Check sheet for the modelled part. Datum: model origin and axes. Units: mm. A direction names the side the tool comes from. Coordinates: 2 decimals unless noted, no trailing zeros. Loops run counter-clockwise (first coordinate to the right, second up) from the corner with the lowest first, then second, coordinate; pieces in that order, holes last. Notation, with made-up numbers: (22.5, 77.25) - (53.5, 77.25) arc R11 ccw to (53.5, 95.25) - close; hole circle Ø4 at (-32.5, -22.75). An arc over 180 degrees is marked (long way). Use a Markdown table: item, result. Add a question column.
1) Thickness scan on line 1 (X direction, y = -1.6, z = 0); line 2 (Y direction, x = 12.5, z = -28); line 3 (X direction, y = -7.5, z = -47.5). Record the ranges inside material, lowest first.
2) Go/stop test with flat-tipped pins: P1, Ø1.5, axis at y = -9, z = 35.5, coming from the -X side; P2, Ø15, axis at x = 4.5, z = -7.5, coming from the +Y side; P3, Ø2, axis at x = 0, z = -31, coming from the -Y side; P4, Ø3, axis at x = -3, z = -26.5, coming from the +Y side. Record where each tip stops, or that it passes through.
3) Draft check along X on faces 4 (the cylindrical face through (52.5, -6.4, 0.1)), 5 (the flat face through (0, -4.555, 30)), 6 (the flat face through (43, -6, -5)). Enter one of: pulls with the +X half, pulls with the -X half, needs draft (parallel to the pull), parting line crosses it, or undercut.
4) Sectioned sample at A-A, the plane y = -7.5. State how many separate pieces and enclosed holes the cut face has, then the cut area to 3 significant figures.
5) Sectioned sample at B-B, the plane x = -30. Enter the section's corners in (y, z).
6) Sectioned sample at C-C, the plane z = -30. Enter the section's corners in (x, y).
7) Tool access check on faces 1 (the flat face through (5, -6, -43)), 2 (the flat face through (24.5, -1.955, -7.8)), 3 (the flat face through (-43, -6, -5)). Record the directions out of +Z, -Z, +X, -X, +Y, -Y that give a thin tool (end or side, any length) a straight path to the whole face; none if there is none.
from build123d import *

# Parameters (mm, degrees)
SKETCH2_R           = 2.15
BOSS_EXTRUDE1_DEPTH = 10.507214
CUT_EXTRUDE2_DEPTH  = 7
SKETCH4_R           = 2.15
CUT_EXTRUDE3_DEPTH  = 7
BOSS_EXTRUDE2_START = -7
SKETCH5_R           = 24.3
SKETCH5_R_2         = 23.3
BOSS_EXTRUDE2_DEPTH = 7
SKETCH6_R           = 23.3
CUT_EXTRUDE4_DEPTH  = 75.575465


with BuildPart() as part:
    # Sketch1 → Revolve1 (revolve)
    with BuildSketch(Plane(origin=(0, 0, 0), x_dir=(0, 0, -1), z_dir=(1, 0, 0)), mode=Mode.PRIVATE) as revolve1_sk:
        with BuildLine():
            Line((-37.5, -1.048229), (-37.5, -1.955443))
            Line((-37.5, -1.955443), (-25.3, -1.955443))
            ThreePointArc((-25.3, -1.955443), (-25, -2.455443), (-25.3, -2.955443))
            Line((-25.3, -2.955443), (-25.3, -4.555443))
            Line((-25.3, -4.555443), (-8, -4.555443))
            Line((-8, -4.555443), (-8, -11.555443))
            Line((-8, -11.555443), (-39.5, -11.555443))
            Line((-39.5, -11.555443), (-39.5, -1.048229))
            Line((-39.5, -1.048229), (-37.5, -1.048229))
        make_face()
    revolve(revolve1_sk.sketch.rotate(Axis((0, -1000, 0), (0, 1, 0)), 180), axis=Axis((0, -1000, 0), (0, 1, 0)))

    # Sketch2 → Boss-Extrude1 (add)
    # profile 1 of 4: a face of its own
    with BuildSketch(Plane.XZ.offset(11.555443)):
        with BuildLine():
            Line((-5, 47.5), (-5, 39.182266))
            Line((-5, 39.182266), (5, 39.182266))
            Line((5, 39.182266), (5, 47.5))
            ThreePointArc((5, 47.5), (0, 52.5), (-5, 47.5))
        make_face()
        with Locations(Location((0, 47.5, 0), (0, 0, 270))):
            Circle(SKETCH2_R, mode=Mode.SUBTRACT)
    # profile 2 of 4: a face of its own
    with BuildSketch(Plane.XZ.offset(11.555443)):
        with BuildLine():
            Line((47.5, -5), (39.182266, -5))
            Line((39.182266, -5), (39.182266, 5))
            Line((39.182266, 5), (47.5, 5))
            ThreePointArc((47.5, 5), (52.5, 0), (47.5, -5))
        make_face()
        with Locations(Location((47.5, 0, 0), (0, 0, 270))):
            Circle(SKETCH2_R, mode=Mode.SUBTRACT)
    # profile 3 of 4: a face of its own
    with BuildSketch(Plane.XZ.offset(11.555443)):
        with BuildLine():
            Line((-5, -47.5), (-5, -39.182266))
            Line((-5, -39.182266), (5, -39.182266))
            Line((5, -39.182266), (5, -47.5))
            ThreePointArc((5, -47.5), (0, -52.5), (-5, -47.5))
        make_face()
        with Locations(Location((0, -47.5, 0), (0, 0, 270))):
            Circle(SKETCH2_R, mode=Mode.SUBTRACT)
    # profile 4 of 4: a face of its own
    with BuildSketch(Plane.XZ.offset(11.555443)):
        with BuildLine():
            Line((-47.5, 5), (-39.182266, 5))
            Line((-39.182266, 5), (-39.182266, -5))
            Line((-39.182266, -5), (-47.5, -5))
            ThreePointArc((-47.5, -5), (-52.5, 0), (-47.5, 5))
        make_face()
        with Locations(Location((-47.5, 0, 0), (0, 0, 270))):
            Circle(SKETCH2_R, mode=Mode.SUBTRACT)
    extrude(amount=-BOSS_EXTRUDE1_DEPTH)

    # Sketch3 → Cut-Extrude2 (cut)
    with BuildSketch(Plane(origin=(0, -4.555443, 0), x_dir=(1, 0, 0), z_dir=(0, 1, 0))):
        with BuildLine():
            Line((21.938323, -2), (12.369317, -2))
            ThreePointArc((12.369317, -2), (11.19262, -2.382785), (10.466345, -3.384615))
            ThreePointArc((10.466345, -3.384615), (7.778175, -7.778175), (3.384615, -10.466345))
            ThreePointArc((3.384615, -10.466345), (2.382785, -11.19262), (2, -12.369317))
            Line((2, -12.369317), (2, -21.938323))
            ThreePointArc((2, -21.938323), (2.718885, -23.474143), (4.358744, -23.905885))
            ThreePointArc((4.358744, -23.905885), (17.182695, -17.182695), (23.905885, -4.358744))
            ThreePointArc((23.905885, -4.358744), (23.474143, -2.718885), (21.938323, -2))
        make_face()
        with BuildLine():
            Line((-2, -21.938323), (-2, -12.369317))
            ThreePointArc((-2, -12.369317), (-2.382785, -11.19262), (-3.384615, -10.466345))
            ThreePointArc((-3.384615, -10.466345), (-7.778175, -7.778175), (-10.466345, -3.384615))
            ThreePointArc((-10.466345, -3.384615), (-11.19262, -2.382785), (-12.369317, -2))
            Line((-12.369317, -2), (-21.938323, -2))
            ThreePointArc((-21.938323, -2), (-23.474143, -2.718885), (-23.905885, -4.358744))
            ThreePointArc((-23.905885, -4.358744), (-17.182695, -17.182695), (-4.358744, -23.905885))
            ThreePointArc((-4.358744, -23.905885), (-2.718885, -23.474143), (-2, -21.938323))
        make_face()
        with BuildLine():
            Line((-21.938323, 2), (-12.369317, 2))
            ThreePointArc((-12.369317, 2), (-11.19262, 2.382785), (-10.466345, 3.384615))
            ThreePointArc((-10.466345, 3.384615), (-7.778175, 7.778175), (-3.384615, 10.466345))
            ThreePointArc((-3.384615, 10.466345), (-2.382785, 11.19262), (-2, 12.369317))
            Line((-2, 12.369317), (-2, 21.938323))
            ThreePointArc((-2, 21.938323), (-2.718885, 23.474143), (-4.358744, 23.905885))
            ThreePointArc((-4.358744, 23.905885), (-17.182695, 17.182695), (-23.905885, 4.358744))
            ThreePointArc((-23.905885, 4.358744), (-23.474143, 2.718885), (-21.938323, 2))
        make_face()
        with BuildLine():
            Line((2, 21.938323), (2, 12.369317))
            ThreePointArc((2, 12.369317), (2.382785, 11.19262), (3.384615, 10.466345))
            ThreePointArc((3.384615, 10.466345), (7.778175, 7.778175), (10.466345, 3.384615))
            ThreePointArc((10.466345, 3.384615), (11.19262, 2.382785), (12.369317, 2))
            Line((12.369317, 2), (21.938323, 2))
            ThreePointArc((21.938323, 2), (23.474143, 2.718885), (23.905885, 4.358744))
            ThreePointArc((23.905885, 4.358744), (17.182695, 17.182695), (4.358744, 23.905885))
            ThreePointArc((4.358744, 23.905885), (2.718885, 23.474143), (2, 21.938323))
        make_face()
    extrude(amount=-CUT_EXTRUDE2_DEPTH, mode=Mode.SUBTRACT)

    # Sketch4 → Cut-Extrude3 (cut)
    with BuildSketch(Plane(origin=(0, -11.555443, 0), x_dir=(-1, 0, 0), z_dir=(0, -1, 0))):
        with Locations(Location((30, 0, 0), (0, 0, 90))):
            Circle(SKETCH4_R)
        with Locations(Location((0, -30, 0), (0, 0, 90))):
            Circle(SKETCH4_R)
        with Locations(Location((-30, 0, 0), (0, 0, 90))):
            Circle(SKETCH4_R)
        with Locations(Location((0, 30, 0), (0, 0, 90))):
            Circle(SKETCH4_R)
    extrude(amount=-CUT_EXTRUDE3_DEPTH, mode=Mode.SUBTRACT)

    # Sketch5 → Boss-Extrude2 (add)
    with BuildSketch(Plane.XZ.offset(11.555443).offset(BOSS_EXTRUDE2_START)):
        Circle(SKETCH5_R)
        Circle(SKETCH5_R_2, mode=Mode.SUBTRACT)
    extrude(amount=BOSS_EXTRUDE2_DEPTH)

    # Sketch6 → Cut-Extrude4 (cut, through all)
    with BuildSketch(Plane(origin=(0, -4.555443, 0), x_dir=(1, 0, 0), z_dir=(0, 1, 0))):
        with Locations(Location((0, 0, 0), (0, 0, 90))):
            Circle(SKETCH6_R)
    extrude(amount=-CUT_EXTRUDE4_DEPTH, mode=Mode.SUBTRACT)


solid = part.part
Solved:
| question | item | result |
|---|---|---|
| 1 | line 1 | x = -52.5 to -49.65, -45.35 to -37.5, 37.5 to 45.35, 49.65 to 52.5 |
| 1 | line 2 | y = -11.56 to -1.96 |
| 1 | line 3 | x = -5 to -2.15, 2.15 to 5 |
| 2 | P1 | stops at x = -18.78 |
| 2 | P2 | passes through |
| 2 | P3 | stops at y = -4.56 |
| 2 | P4 | stops at y = -1.96 |
| 3 | face 4 | pulls with the +X half |
| 3 | face 5 | undercut |
| 3 | face 6 | needs draft |
| 4 | separate pieces | 1 |
| 4 | enclosed holes | 9 |
| 4 | area | 3,560 mm2 |
| 5 | outline | (-11.56, -25.7) - (-1.05, -25.7) - (-1.05, -22.5) - (-1.96, -22.5) - (-1.96, 22.5) - (-1.05, 22.5) - (-1.05, 25.7) - (-11.56, 25.7) - (-11.56, 2.15) - (-4.56, 2.15) - (-4.56, -2.15) - (-11.56, -2.15) - close |
| 6 | outline | (-25.7, -11.56) - (-2.15, -11.56) - (-2.15, -4.56) - (2.15, -4.56) - (2.15, -11.56) - (25.7, -11.56) - (25.7, -1.05) - (22.5, -1.05) - (22.5, -1.96) - (-22.5, -1.96) - (-22.5, -1.05) - (-25.7, -1.05) - close |
| 7 | face 1 | -Z, +X, +Y, -Y |
| 7 | face 2 | +Y |
| 7 | face 3 | -Z, -X, +Y, -Y |
